```python
from build123d import *

# Parameters (mm, degrees)
F1_DEPTH = 45
F2_R     = 4.99999
F3_R     = 9.5
F4_DEPTH = 80


# Not quite as in the source:
# - a fillet or chamfer is up to 0.001 mm smaller than in the source, because OpenCascade refuses the exact size


with BuildPart() as f1:
    # F0 (on Top) → F1 (new body)
    with BuildSketch(Plane.XY):
        Polygon((65.8763971276, 17.5545628369), (-34.1236028724, 17.5545628369), (-34.1236028724, 12.5545628369), (60.8763971276, 12.5545628369), (60.8763971276, -27.4454371631), (-34.1236028724, -27.4454371631), (-34.1236028724, -32.4454371631), (-34.1236028724, -37.4454371631), (-29.1236028724, -37.4454371631), (-29.1236028724, -32.4454371631), (60.8763971276, -32.4454371631), (60.8763971276, -37.4454371631), (65.8763971276, -37.4454371631), (65.8763971276, -32.4454371631), align=None)
    extrude(amount=F1_DEPTH)

    # F2 (radius 5 in the source; OpenCascade refuses exactly that, so slightly less here)
    f2_edges = [f1.edges().sort_by_distance(p)[0] for p in [
        (60.876397, 12.554563, 22.5),
        (60.876397, -27.445437, 22.5),
        (65.876397, 17.554563, 22.5),
        (60.876397, -32.445437, 22.5),
        (-29.123603, -32.445437, 22.5),
        (-34.123603, -27.445437, 22.5),
    ]]
    fillet(f2_edges, radius=F2_R)

    # F3 (on face) → F4 (cut)
    with BuildSketch(Plane(origin=(0, 17.5545628369, 0), x_dir=(-1, 0, 0), z_dir=(0, 1, 0))):
        with Locations((-45.8763971276, 33)):
            Circle(F3_R)
        with Locations((-0.8763971276, 12)):
            Circle(F3_R)
        with Locations((14.1236028724, 33)):
            Circle(F3_R)
        with Locations((-30.8763971276, 12)):
            Circle(F3_R)
        with Locations((-15.8763971276, 33)):
            Circle(F3_R)
    extrude(amount=-F4_DEPTH, mode=Mode.SUBTRACT)


solid = f1.part
```
Check sheet for the modelled part. Datum: model origin and axes. Units: mm. A direction names the side the tool comes from. Round coordinates to 2 decimals unless told otherwise and drop trailing zeros. Loops run counter-clockwise (first coordinate to the right, second up) from the corner with the lowest first, then second, coordinate; pieces in that order, holes last. Notation, with made-up numbers: (86.5, -40) - (135.5, -40) arc R7 ccw to (135.5, -30) - close; hole circle Ø11 at (-31, 72.25). An arc over 180 degrees is marked (long way). Write item = value, one per line. Start each with the question number.
Q1. Section check B-B (x = -3.5). Record the boundary of the cut face in (y, z), plus the area to 3 significant figures.
Q2. Section check A-A (z = 12). Count the separate pieces of the cut face and the enclosed holes in it, plus the area to 3 significant figures.
Q3. Section check C-C (y = -29). Record the boundary of the cut face in (x, z), plus the area to 3 significant figures.
Q4. Depth check by flat-ended pin: P1, Ø17, axis at x = 45.88, z = 33, coming from the -Y side; P2, Ø22, axis at x = 15.88, z = 33, coming from the +Y side; P3, Ø22.5, axis at x = 7, z = 31, coming from the -Y side. Enter the tip coordinate at first touch or a pass-through.
Q5. Access from +Z, -Z, +X, -X, +Y, -Y to the whole of each face (thin tool, end or side, straight path). Record for faces 4 (the face through (59.4, 11.1, 22.8)), 5 (the face through (15, -32.445, 22)), 6 (the face through (-19.23, 15.09, 41.01)).
Q6. Release check for a two-part mould opening along Y. For faces 1 (the face through (-34.124, 15, 22)), 2 (the face through (-32, -37.445, 22)), 3 (the face through (-32.62, -28.87, 22.82)) record: pulls with the +Y half, pulls with the -Y half, needs draft (parallel to the pull), parting line crosses it, or undercut.
Q7. Thickness scan on L1, parallel to Y at x = -29.5, z = 43; L2, parallel to Y at x = -3, z = 41.5; L3, parallel to X at y = -4, z = 5.5. Record the ranges inside material, lowest first.
Derived:
q1.outline = (-32.45, 0) - (-27.45, 0) - (-27.45, 3.57) - (-32.45, 3.57) - close; (-32.45, 20.43) - (-27.45, 20.43) - (-27.45, 45) - (-32.45, 45) - close; (12.55, 0) - (17.55, 0) - (17.55, 3.57) - (12.55, 3.57) - close; (12.55, 20.43) - (17.55, 20.43) - (17.55, 45) - (12.55, 45) - close
q1.area = 281 mm^2
q2.separate_pieces = 5
q2.enclosed_holes = 0
q2.area = 881 mm^2
q3.outline = (-32.75, 0) - (65.88, 0) - (65.88, 45) - (-32.75, 45) - close; hole circle Ø19 at (-14.12, 33); hole circle Ø19 at (0.88, 12); hole circle Ø19 at (15.88, 33); hole circle Ø19 at (30.88, 12); hole circle Ø19 at (45.88, 33)
q3.area = 3,020 mm^2
q4.P1 = through
q4.P2 = 17.55
q4.P3 = -32.45
q5.face_4 = +Z, -Z, -X
q5.face_5 = +Z, -Z, -Y
q5.face_6 = +Y, -Y
q6.face_1 = needs draft
q6.face_2 = pulls with the -Y half
q6.face_3 = undercut
q7.L1 = -37.45 to -27.46, 12.55 to 17.55
q7.L2 = -32.45 to -27.45, 12.55 to 17.55
q7.L3 = 60.88 to 65.88
